For this review, take the finished solid that the model builds, in its own axes (mm). A direction names the side the tool comes from. Give positions to 0.01 mm unless a question says otherwise; leave off trailing zeros. Write each loop counter-clockwise with the first axis right and the second up, starting at its lowest first coordinate (ties: lowest second). Pieces come first, ordered by that corner, then holes.
1) We need section D-D on y = 3.25. Give the boundary of the cut face in (x, z), and give its area (3 significant figures).
2) Draft analysis for pull direction X (two halves, no side actions). For faces 3 (the face through (0, 4.9, -1.5)), 4 (the face through (-1.05, 4.44, -0.33)), 5 (the face through (-2.1, 4.82, 0.97)), 6 (the face through (-1.5, 4.9, 0)), state which applies: pulls with the +X half, pulls with the -X half, needs draft (parallel to the pull), parting line crosses it, or undercut.
3) For P1, Ø1, axis at y = 3, z = -1.5, coming from the -X side; P2, Ø1.5, axis at x = 1.5, y = 8, coming from the -Z side; P3, Ø0.8, axis at x = -1.5, y = 4.5, coming from the +Z side, all flat-tipped, find the tip position at first contact; note any pin that passes through.
4) We need section A-A on z = 2.1. Give the boundary of the cut face in (x, y), and give its area (3 significant figures).
5) Machinability: for faces 1 (the face through (-1, 9, -1)), 2 (the face through (0.97, 4.98, -2.1)), which of the approach directions +Z, -Z, +X, -X, +Y, -Y give a long, thin tool a straight path to every point of the face, cutting with its end or side? Answer none if there is none.
6) We need section C-C on y = 0.75. Give the boundary of the cut face in (x, z).
7) We need section B-B on z = 1. Give the boundary of the cut face in (x, y).
8) Wall thickness on line 1 along Z through (x, y) = (0, 2.75); line 2 along Y through (x, z) = (0, 1.35); line 3 along Z through (x, y) = (2.3, 1.75): over which ranges is each line inside the solid? List them lowest first.
Autodesk Inventor part; units mm, degrees
ref_plane "YZ Plane" through (0, 0, 0) normal (1, 0, 0) x (0, 1, 0)
ref_plane "XZ Plane" through (0, 0, 0) normal (0, 1, 0) x (-1, 0, 0)
ref_plane "XY Plane" through (0, 0, 0) normal (0, 0, 1) x (1, 0, 0)
sketch "Sketch1" plane through (0, 0, 0) normal (0, 1, 0) x (-1, 0, 0)
  circle A0 centre (0, 0) radius 1.1
  circle A1 centre (0, 0) radius 2.55
  dimension "d0" = 2.2
  dimension "d1" = 5.1
extrude "Extrusion1" add sketch "Sketch1" along normal blind 9
sketch "Sketch2" plane through (0, 0, 0) normal (0, 0, 1) x (1, 0, 0)
  line L0 (2.55, 9) -> (-2.55, 9)
  line L1 (2.55, 0) -> (-2.55, 0)
  line L2 (-2.55, 0) -> (-2.55, 9)
  line L3 (-2.55, 7) -> (2.5173, 7)
  line L4 (2.55, 9) -> (-2.55, 9)
  line L5 (0, 9) -> (0, 0)
  circle A0 centre (0, 4.9) radius 2.1
  dimension "d4" = 2
  dimension "d5" = 4.2
extrude "Extrusion2" cut sketch "Sketch2" along normal blind 12 contours A0 L5 | L5 A0
sketch "Sketch3" plane through (0, 0, 0) normal (1, 0, 0) x (0, 1, 0)
  line L0 (9, -2.55) -> (9, 2.55)
  line L1 (0, -2.55) -> (0, 2.55)
  line L2 (0, 2.55) -> (9, 2.55)
  line L3 (7, 2.55) -> (7, -2.525)
  line L4 (9, 1.1) -> (9, -1.1)
  line L5 (9, 0) -> (0, 0)
  circle A0 centre (4.9, 0) radius 2.1
  point P0 (4.9, 1.4465)
  dimension "d8" = 2
  dimension "d9" = 4.2
extrude "Extrusion3" cut sketch "Sketch3" along normal up to next contours A0 L5 | L5 A0
properties part number "motor_shaft_adapter" material "ABS Plastic"
Results list:
1. outline: (-1.3, 0) - (-1.3, 2.19) arc R2.55 ccw (long way) to (2.19, -1.3) - (0, -1.3) - (0, -1.1) arc R1.1 cw to (-1.1, 0) - close; (1.3, 1.3) - (2.19, 1.3) arc R2.55 ccw to (1.3, 2.19) - close
1. area: 8.51 mm2
2. face 3: pulls with the +X half
2. face 4: undercut
2. face 5: undercut
2. face 6: needs draft
3. P1: stops at x = -2.35
3. P2: stops at z = -2.44
3. P3: stops at z = 0
4. outline: (-1.45, 0) - (1.45, 0) - (1.45, 3.38) arc R2.1 cw to (-1.45, 3.38) - close; (-1.45, 6.42) arc R2.1 cw to (1.45, 6.42) - (1.45, 9) - (-1.45, 9) - close
4. area: 14.9 mm2
5. face 1: +Z, -Z, +X, -X, +Y
5. face 2: +X
6. outline: circle Ø5.1 at (0, 0); hole circle Ø2.2 at (0, 0)
7. outline: (-2.35, 0) - (-0.46, 0) - (-0.46, 2.85) arc R2.1 cw to (-0.46, 6.95) - (-0.46, 9) - (-2.35, 9) - close; (0.46, 0) - (2.35, 0) - (2.35, 3.05) - (1, 3.05) arc R2.1 cw to (0.46, 2.85) - close; (0.46, 6.95) arc R2.1 cw to (1, 6.75) - (2.35, 6.75) - (2.35, 9) - (0.46, 9) - close
8. line 1: z = -2.55 to -1.1, 1.1 to 2.55
8. line 2: y = 0 to 2.8, 7 to 9
8. line 3: z = -1.1 to 1.1
